Work out the finished part from the listing and answer in its coordinate system (mm). Face numbers are marked on the shaded views. A direction names the side the tool comes from. Coordinates: 2 decimals unless noted, no trailing zeros. Order: outer loops, then holes, each group sorted by start corner. A loop starts at its lowest first (then second) coordinate and runs counter-clockwise, first axis right, second up. Notation, with made-up numbers: (-17, 81) -> (34, 81) arc R28 ccw to (34, 112) -> close; hole circle Ø6 at (-7, -26.75). An arc over 180 degrees is marked (long way). Answer as CSV lines item,"result". Start each with the question number.
Item 1: Section A-A (y = 0) is taken. Write down the section's boundary in (x, z) (3 decimals).
Item 2: For a pull along Y with two mould halves and no side action, classify the marked faces 3, 4 and 5 as pulls with the +Y half, pulls with the -Y half, needs draft (parallel to the pull), parting line crosses it, or undercut.
Item 3: Section D-D (y = -51) is taken. Write down the section's boundary in (x, z).
Item 4: Section B-B (x = 0) is taken. Write down the section's boundary in (y, z) (3 decimals), then the cut area to 3 significant figures.
Item 5: Which of the six approach directions +Z, -Z, +X, -X, +Y, -Y give full straight-line access (tool end or side, diameter ignored) to the marked faces 1 and 2?
Item 6: This flat-tipped pin is pushed along its axis until it touches: pin 1 Ø10 at (x, y) = (-13.5, -53) entering from +Z. Where does it stop, or does it pass through?
Item 7: Straight lines are drawn through the part: L1, parallel to Y at x = 0, z = 10.75; L2, parallel to X at y = 0, z = 4.5 (3 decimals); L3, parallel to Z at x = 18.5, y = -59.5. For each, find the intervals that lie inside material, in ascending order.
Item 8: Section C-C (z = 15.75) is taken. Write down the section's boundary in (x, y).
```python
from build123d import *

# Parameters (mm, degrees)
BOSS_EXTRUDE1_DEPTH = 6.35
SKETCH2_W           = 152.4
SKETCH2_H           = 142.24
SKETCH2_R           = 58.42
BOSS_EXTRUDE2_DEPTH = 11.43


with BuildPart() as part:
    # Sketch1 → Boss-Extrude1 (new body)
    with BuildSketch(Plane.XY):
        with BuildLine():
            Line((-31.75, 71.12), (-76.2, 71.12))
            Line((-76.2, 71.12), (-76.2, -71.12))
            Line((-76.2, -71.12), (76.2, -71.12))
            Line((76.2, -71.12), (76.2, 71.12))
            Line((76.2, 71.12), (31.75, 71.12))
            Line((31.75, 71.12), (31.75, 58.630138368))
            ThreePointArc((31.75, 58.630138368), (0, -66.675), (-31.75, 58.630138368))
            Line((-31.75, 58.630138368), (-31.75, 71.12))
        make_face()
    extrude(amount=BOSS_EXTRUDE1_DEPTH)

    # Sketch2 → Boss-Extrude2 (add)
    with BuildSketch(Plane.XY.offset(6.35)):
        Rectangle(SKETCH2_W, SKETCH2_H)
        Circle(SKETCH2_R, mode=Mode.SUBTRACT)
    extrude(amount=BOSS_EXTRUDE2_DEPTH)


solid = part.part
```
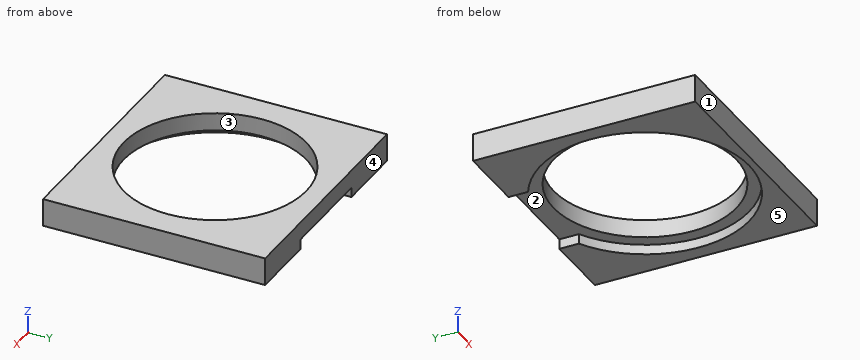
Checked values:
1,outline,"(-76.2, 0) -> (-66.675, 0) -> (-66.675, 6.35) -> (-58.42, 6.35) -> (-58.42, 17.78) -> (-76.2, 17.78) -> close; (58.42, 6.35) -> (66.675, 6.35) -> (66.675, 0) -> (76.2, 0) -> (76.2, 17.78) -> (58.42, 17.78) -> close"
2,face 3,"undercut"
2,face 4,"pulls with the +Y half"
2,face 5,"needs draft"
3,outline,"(-76.2, 0) -> (-42.95, 0) -> (-42.95, 6.35) -> (-28.49, 6.35) -> (-28.49, 17.78) -> (-76.2, 17.78) -> close; (28.49, 6.35) -> (42.95, 6.35) -> (42.95, 0) -> (76.2, 0) -> (76.2, 17.78) -> (28.49, 17.78) -> close"
4,outline,"(-71.12, 0) -> (-66.675, 0) -> (-66.675, 6.35) -> (-58.42, 6.35) -> (-58.42, 17.78) -> (-71.12, 17.78) -> close; (58.42, 6.35) -> (71.12, 6.35) -> (71.12, 17.78) -> (58.42, 17.78) -> close"
4,area,"319 mm^2"
5,face 1,"+Z, -Z, +X, -X, -Y"
5,face 2,"-Z"
6,pin 1,"stops at z = 17.78"
7,L1,"y = -71.12 to -58.42, 58.42 to 71.12"
7,L2,"x = -76.2 to -66.675, 66.675 to 76.2"
7,L3,"z = 6.35 to 17.78"
8,outline,"(-76.2, -71.12) -> (76.2, -71.12) -> (76.2, 71.12) -> (-76.2, 71.12) -> close; hole circle Ø116.84 at (0, 0)"
